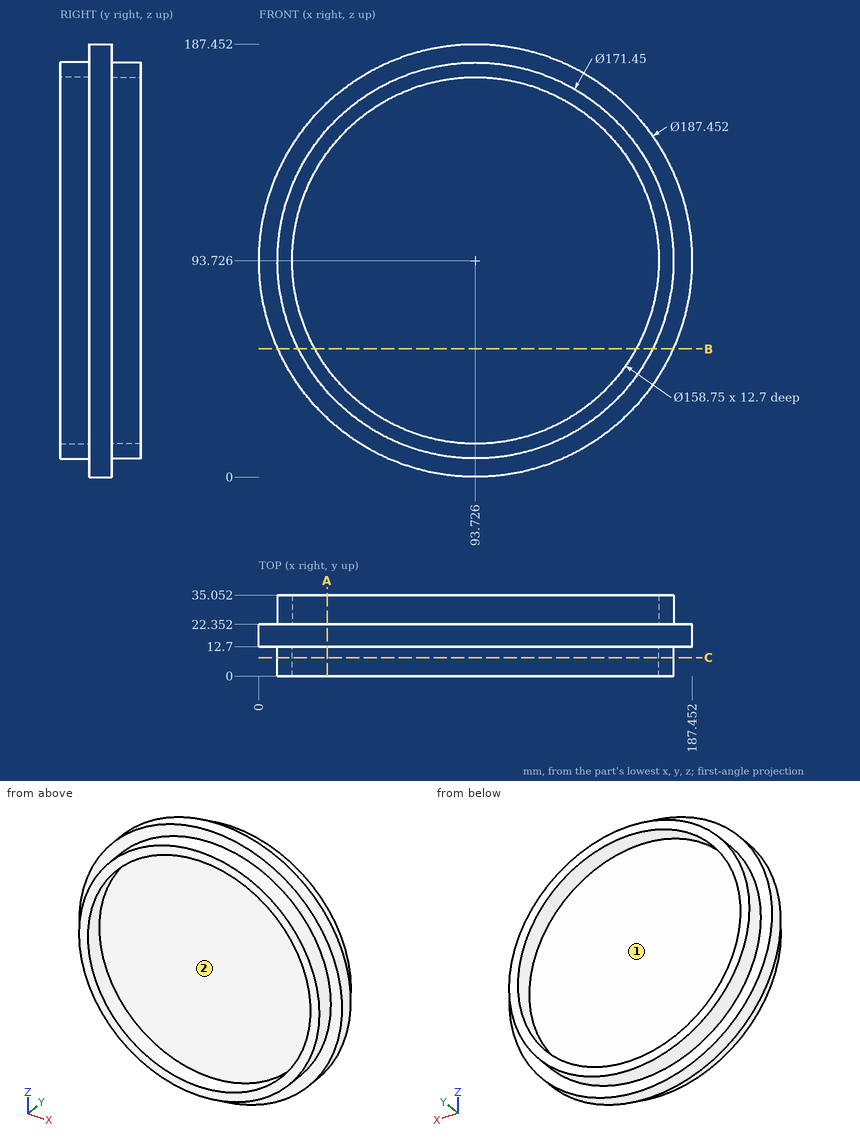
Print and shaded views of the part. All mm, measured from the part's lowest x, y and z. A direction names the side the tool comes from. Coordinates: 2 decimals unless noted, no trailing zeros. Write each loop counter-clockwise with the first axis right and the second up, starting at its lowest first coordinate (ties: lowest second). Pieces come first, ordered by that corner, then holes. Notation, with made-up numbers: (18.5, -23.75) - (44.5, -23.75) arc R29 cw to (44.5, 0.25) - close; hole circle Ø8 at (-19, 40). An arc over 180 degrees is marked (long way). One line per question, with ' | ' between items. Start each with the question number.
Q1. Pin check, flat tips, straight feed: pin 1 (4 mm diameter, centred on y = 17.5, z = 82, fed in from -X); pin 2 (5 mm diameter, centred on y = 29, z = 83, fed in from -X); pin 3 (4 mm diameter, centred on x = 39.5, z = 134.5, fed in from -Y). Stop position of each tip, or through.
Q2. Cut at A-A, the plane x = 29.5. List the corners of the cut face in (y, z).
Q3. 3-axis set-ups, long thin cutter, end or side, ignore diameter. For the marked faces 1 and 2: which of +Z, -Z, +X, -X, +Y, -Y reach the whole face in a straight line?
Q4. Cut at C-C, the plane y = 8. List the corners of the cut face in (x, z) (3 decimals), then the cut area to 3 significant figures.
Q5. Cut at B-B, the plane z = 55.5. List the corners of the cut face in (x, y), then the cut area to 3 significant figures.
Q6. Drill centre lines: line 1 (Z direction, x = 114, y = 8.5); line 2 (Y direction, x = 136, z = 137); line 3 (X direction, y = 7, z = 84.5). Where is each one in solid material? Low to high. Write a range as [from, to].
Answer below:
1) pin 1: x = 0.51 | pin 2: x = 8.4 | pin 3: y = 12.7
2) outline: (0, 36.95) - (12.7, 36.95) - (12.7, 25.46) - (22.35, 25.46) - (22.35, 36.95) - (35.05, 36.95) - (35.05, 47.08) - (22.35, 47.08) - (22.35, 140.37) - (35.05, 140.37) - (35.05, 150.5) - (22.35, 150.5) - (22.35, 161.99) - (12.7, 161.99) - (12.7, 150.5) - (0, 150.5) - (0, 140.37) - (12.7, 140.37) - (12.7, 47.08) - (0, 47.08) - close
3) face 1: +Y | face 2: -Y
4) outline: circle Ø171.45 at (93.726, 93.726); hole circle Ø158.75 at (93.726, 93.726) | area: 3,290 mm^2
5) outline: (8.15, 12.7) - (17, 12.7) - (17, 0) - (24.16, 0) - (24.16, 12.7) - (163.29, 12.7) - (163.29, 0) - (170.46, 0) - (170.46, 12.7) - (179.3, 12.7) - (179.3, 22.35) - (170.46, 22.35) - (170.46, 35.05) - (163.29, 35.05) - (163.29, 22.35) - (24.16, 22.35) - (24.16, 35.05) - (17, 35.05) - (17, 22.35) - (8.15, 22.35) - close | area: 2,020 mm^2
6) line 1: [10.43, 16.98], [170.47, 177.02] | line 2: [12.7, 22.35] | line 3: [8.5, 14.89], [172.56, 178.95]
